from build123d import *

# Parameters (mm, degrees)
BOSS_EXTRU_1_DEPTH           = 5
BOSS_EXTRU_2_DEPTH           = 2
SYM_TRIE2_COPY_1_DEPTH       = 2
CONG_1_R                     = 0.5
ESQUISSE4_R                  = 1.5
ENL_V_MAT_EXTRU_2_DEPTH      = 1.0000001
ENL_V_MAT_EXTRU_2_DEPTH_BACK = 11.0000001
ESQUISSE5_R                  = 1
ENL_V_MAT_EXTRU_3_DEPTH      = 7
ESQUISSE3_R                  = 1
ENL_V_MAT_EXTRU_1_DEPTH      = 14.500000115
ENL_V_MAT_EXTRU_1_DEPTH_BACK = 4


with BuildPart() as part:
    # Esquisse1 → Boss.-Extru.1 (new body, symmetric)
    with BuildSketch(Plane.XY):
        with BuildLine():
            Line((-20, 0), (20, 0))
            Line((20, 0), (20, 3))
            Line((20, 3), (7.5, 3))
            Line((7.5, 3), (7.5, 9))
            ThreePointArc((7.5, 9), (0, 16.5), (-7.5, 9))
            Line((-7.5, 9), (-7.5, 3))
            Line((-7.5, 3), (-20, 3))
            Line((-20, 3), (-20, 0))
        make_face()
    extrude(amount=BOSS_EXTRU_1_DEPTH, both=True)

    # Esquisse2 → Boss.-Extru.2 (add)
    with BuildSketch(Plane.XY.offset(5)):
        Polygon((-10.5, 3), (-7.5, 6), (-7.5, 3), align=None)
    boss_extru_2 = extrude(amount=-BOSS_EXTRU_2_DEPTH)

    # Symétrie1: Boss.-Extru.2 across plane
    add(boss_extru_2.mirror(Plane.XY))

    # Symétrie2: Boss.-Extru.2 across plane
    add(boss_extru_2.mirror(Plane(origin=(0, 0, 0), x_dir=(0, 0, 1), z_dir=(1, 0, 0))))

    # Symétrie2 copy 1 sketch → Symétrie2 copy 1 (add)
    with BuildSketch(Plane(origin=(0, 0, -5), x_dir=(-1, 0, 0), z_dir=(0, 0, -1))):
        Polygon((-10.5, 3), (-7.5, 6), (-7.5, 3), align=None)
    extrude(amount=-SYM_TRIE2_COPY_1_DEPTH)

    # Congé1
    cong_1_edges = [part.edges().sort_by_distance(p)[0] for p in [
        (20, 1.5, 5),
        (15.25, 3, 5),
        (-20, 3, 0),
        (20, 3, 0),
        (0, 16.5, 5),
        (-7.5, 7.5, 5),
        (-15.25, 3, 5),
        (-9, 4.5, 5),
        (-15.25, 3, -5),
        (-9, 4.5, -5),
        (7.5, 7.5, -5),
        (9, 4.5, -5),
        (7.5, 7.5, 5),
        (9, 4.5, 5),
        (-7.5, 7.5, -5),
        (0, 16.5, -5),
        (15.25, 3, -5),
        (20, 1.5, -5),
    ]]
    fillet(cong_1_edges, radius=CONG_1_R)

    # Esquisse4 → Enlèv. mat.-Extru.2 (cut, two sides)
    with BuildSketch(Plane.XY.offset(5)) as enl_v_mat_extru_2_sk:
        with Locations((0, 9)):
            Circle(ESQUISSE4_R)
    extrude(amount=ENL_V_MAT_EXTRU_2_DEPTH, mode=Mode.SUBTRACT)
    extrude(enl_v_mat_extru_2_sk.sketch, amount=-ENL_V_MAT_EXTRU_2_DEPTH_BACK, mode=Mode.SUBTRACT)

    # Esquisse5 → Enlèv. mat.-Extru.3 (cut)
    with BuildSketch(Plane(origin=(0, 16.5, 0), x_dir=(1, 0, 0), z_dir=(0, 1, 0))):
        Circle(ESQUISSE5_R)
    extrude(amount=-ENL_V_MAT_EXTRU_3_DEPTH, mode=Mode.SUBTRACT)

    # Esquisse3 → Enlèv. mat.-Extru.1 (cut, two sides)
    with BuildSketch(Plane(origin=(0, 3, 0), x_dir=(1, 0, 0), z_dir=(0, 1, 0))) as enl_v_mat_extru_1_sk:
        with Locations((-16, 0)):
            Circle(ESQUISSE3_R)
        with Locations((16, 0)):
            Circle(ESQUISSE3_R)
    extrude(amount=ENL_V_MAT_EXTRU_1_DEPTH, mode=Mode.SUBTRACT)
    extrude(enl_v_mat_extru_1_sk.sketch, amount=-ENL_V_MAT_EXTRU_1_DEPTH_BACK, mode=Mode.SUBTRACT)


solid = part.part
Could you check a few things on this model? Use its own coordinates, in mm. A direction names the side the tool comes from. Round coordinates to 2 decimals unless told otherwise and drop trailing zeros. Order: outer loops, then holes, each group sorted by start corner. A loop starts at its lowest first (then second) coordinate and runs counter-clockwise, first axis right, second up.
Q1. Which directions (+Z, -Z, +X, -X, +Y, -Y) give clear straight access to the entire face, cutting with the end or side of a thin tool? Please do faces 4 (the face through (0, 13, 1)), 5 (the face through (-8, 4, 3)), 6 (the face through (8.88, 4.42, -4.85)), 7 (the face through (9, 4.5, 3.8)), 8 (the face through (14, 3, 0)).
Geometry says:
face 4: +Y
face 5: -X, +Y
face 6: -Z, +X, +Y
face 7: +Z, -Z, +X, +Y
face 8: +X, +Y
Q2. Imagine slicing it at C-C, the plane x = -14.5. List the corners of the cut face in (y, z) for me, then the cut area to 3 significant figures.
Geometry says:
outline: (0, -5) - (2.5, -5) arc R0.5 ccw to (3, -4.5) - (3, 4.5) arc R0.5 ccw to (2.5, 5) - (0, 5) - close
area: 29.9 mm2
Q3. Please list where these lines run through material, in increasing order: probe 1 along X at (y, z) = (2.3, 0); probe 2 along Z at (x, y) = (0, 13.5); probe 3 along Y at (x, z) = (9, -2).
Geometry says:
probe 1: x = -20 to -17, -15 to 15, 17 to 20
probe 2: z = -5 to -1, 1 to 5
probe 3: y = 0 to 3
Q4. I'm going to push flat-ended pins straight in: P1, Ø3, axis at y = 7, z = 0, coming from the -X side; P2, Ø2.5, axis at x = 9, y = 4, coming from the -Z side; P3, Ø1.5, axis at x = 6.5, z = 3.5, coming from the +Y side; P4, Ø2.5, axis at x = -14.5, z = -2, coming from the +Y side. Where does each tip first touch, or does it pass through?
Geometry says:
P1: stops at x = -7.5
P2: stops at z = -5
P3: stops at y = 13.82
P4: stops at y = 3
Q5. Thinking about a two-plate mould opening in Z: for faces 1 (the face through (20, 1, 0)), 2 (the face through (-1, 6, 5)), 3 (the face through (17, 2, 0)), which applies, released by +Z, released by -Z, zero draft, split by the parting line, or undercut?
Geometry says:
face 1: zero draft
face 2: released by +Z
face 3: undercut
Q6. Imagine slicing it at A-A, the plane x = 16. List the corners of the cut face in (y, z) for me, then the cut area to 3 significant figures.
Geometry says:
outline: (0, -5) - (2.5, -5) arc R0.5 ccw to (3, -4.5) - (3, -1) - (0, -1) - close; (0, 1) - (3, 1) - (3, 4.5) arc R0.5 ccw to (2.5, 5) - (0, 5) - close
area: 23.9 mm2
Q7. Imagine slicing it at B-B, the plane z = 0. List the corners of the cut face in (x, y) for me, then the cut area to 3 significant figures.
Geometry says:
outline: (-20, 0) - (-17, 0) - (-17, 3) - (-19.5, 3) arc R0.5 ccw to (-20, 2.5) - close; (-15, 0) - (15, 0) - (15, 3) - (7.5, 3) - (7.5, 9) arc R7.5 ccw to (1, 16.43) - (1, 10.12) arc R1.5 cw (long way) to (-1, 10.12) - (-1, 16.43) arc R7.5 ccw to (-7.5, 9) - (-7.5, 3) - (-15, 3) - close; (17, 0) - (20, 0) - (20, 2.5) arc R0.5 ccw to (19.5, 3) - (17, 3) - close
area: 267 mm2
